```python
from build123d import *

# Parameters (mm, degrees)
SKETCH1_W                        = 287
SKETCH1_H                        = 303
BOSS_EXTRUDE1_DEPTH              = 1.5
SKETCH8_W                        = 1.5
SKETCH8_H                        = 303
BOSS_EXTRUDE8_DEPTH              = 20
BOSS_EXTRUDE12_DEPTH             = 1.5
BOSS_EXTRUDE13_DEPTH             = 1.5
BOSS_EXTRUDE14_REACH             = 217.497
BOSS_EXTRUDE14_DIRECTION_2_REACH = 217.497


with BuildPart() as part:
    # Sketch1 → Boss-Extrude1 (new body)
    with BuildSketch(Plane(origin=(0, 0, 0), x_dir=(1, 0, 0), z_dir=(0, 1, 0))):
        Rectangle(SKETCH1_W, SKETCH1_H)
    extrude(amount=BOSS_EXTRUDE1_DEPTH)

    # Sketch8 → Boss-Extrude8 (add)
    with BuildSketch(Plane(origin=(0, 1.5, 0), x_dir=(1, 0, 0), z_dir=(0, 1, 0))):
        with Locations((-142.75, 0)):
            Rectangle(SKETCH8_W, SKETCH8_H)
        with Locations((142.75, 0)):
            Rectangle(SKETCH8_W, SKETCH8_H)
    extrude(amount=BOSS_EXTRUDE8_DEPTH)

    # Sketch12 → Boss-Extrude12 (add)
    with BuildSketch(Plane.ZY.offset(143.5)):
        Polygon((-151.5, 21.5), (-159.325360037, 21.5), (-151.5, 0), align=None)
    extrude(amount=-BOSS_EXTRUDE12_DEPTH)

    # Sketch13 → Boss-Extrude13 (add)
    with BuildSketch(Plane(origin=(143.5, 0, 0), x_dir=(0, 0, -1), z_dir=(1, 0, 0))):
        Polygon((151.5, 0), (151.5, 21.5), (159.325360037, 21.5), align=None)
    extrude(amount=-BOSS_EXTRUDE13_DEPTH)

    # Boss-Extrude14: up to this face of the body (flat: up to its plane)
    boss_extrude14_end = Plane(part.part.faces().sort_by_distance((142, 11.538792752, -2.109985057))[0])
    # Sketch15 → Boss-Extrude14 (add, up to the picked face)
    with BuildSketch(Plane(origin=(0, 0, 0), x_dir=(0, 0, -1), z_dir=(1, 0, 0)), mode=Mode.PRIVATE) as boss_extrude14_sk1:
        with BuildLine():
            Line((151.5, 1.5), (158.340402867, 20.293852416))
            Line((158.340402867, 20.293852416), (159.749941798, 19.780822201))
            Line((159.749941798, 19.780822201), (152.909538931, 0.986969785))
            ThreePointArc((152.909538931, 0.986969785), (152.360364655, 0.271271934), (151.5, 0))
            Line((151.5, 0), (151.5, 1.5))
        make_face()
    boss_extrude14_tool1 = split(extrude(boss_extrude14_sk1.sketch, amount=BOSS_EXTRUDE14_REACH, mode=Mode.PRIVATE), bisect_by=boss_extrude14_end, keep=Keep.BOTH, mode=Mode.PRIVATE)
    add(boss_extrude14_tool1.solids().sort_by(Axis((0, 10.206295, -155.467858), (1, 0, 0)))[0])

    # Boss-Extrude14 direction 2: up to this face of the body (flat: up to its plane)
    boss_extrude14_direction_2_end = Plane(part.part.faces().sort_by_distance((-142, 11.538792752, -2.109985057))[0])
    # Sketch15 → Boss-Extrude14 direction 2 (add, up to the picked face)
    with BuildSketch(Plane(origin=(0, 0, 0), x_dir=(0, 0, -1), z_dir=(1, 0, 0)), mode=Mode.PRIVATE) as boss_extrude14_direction_2_sk1:
        with BuildLine():
            Line((151.5, 1.5), (158.340402867, 20.293852416))
            Line((158.340402867, 20.293852416), (159.749941798, 19.780822201))
            Line((159.749941798, 19.780822201), (152.909538931, 0.986969785))
            ThreePointArc((152.909538931, 0.986969785), (152.360364655, 0.271271934), (151.5, 0))
            Line((151.5, 0), (151.5, 1.5))
        make_face()
    boss_extrude14_direction_2_tool1 = split(extrude(boss_extrude14_direction_2_sk1.sketch, amount=-BOSS_EXTRUDE14_DIRECTION_2_REACH, mode=Mode.PRIVATE), bisect_by=boss_extrude14_direction_2_end, keep=Keep.BOTH, mode=Mode.PRIVATE)
    add(boss_extrude14_direction_2_tool1.solids().sort_by(Axis((0, 10.206295, -155.467858), (-1, 0, 0)))[0])


solid = part.part
```
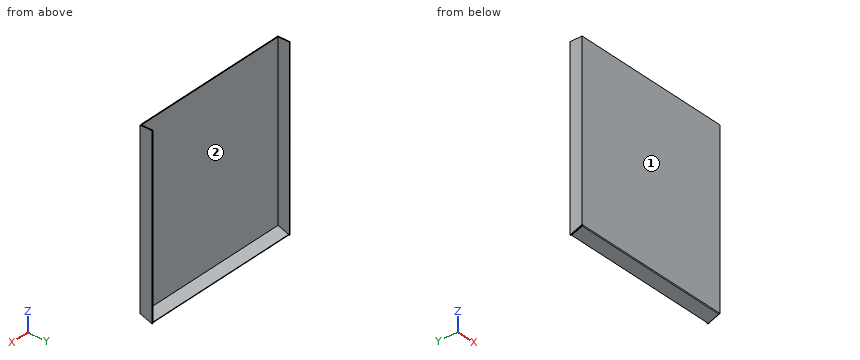
Read the model definition and answer for the solid it produces. Units are mm, in the model's axes. Face numbers are marked on the shaded views. Give positions to 0.01 mm unless a question says otherwise; leave off trailing zeros. Write each loop counter-clockwise with the first axis right and the second up, starting at its lowest first coordinate (ties: lowest second). Pieces come first, ordered by that corner, then holes. Notation, with made-up numbers: (8, 0.5) -> (19, 0.5) arc R21 cw to (19, 32.5) -> close; hole circle Ø5 at (-15.75, 64.25). An arc over 180 degrees is marked (long way). Answer as a JSON object with one key per item and string values.
1) Flat-ended cylindrical pins translate along their axes: pin 1 Ø1 at (x, y) = (-90, 6.5) entering from +Z; pin 2 Ø1.5 at (x, y) = (-101, 15.5) entering from -Z; pin 3 Ø3 at (x, y) = (-34.5, 16) entering from +Z. Find the tip coordinate at first contact, or state that the pin passes through.
Findings below:
{"pin 1": "stops at z = -153.14", "pin 2": "stops at z = -158.46", "pin 3": "stops at z = -156.23"}
2) Section A-A on x = -120.5 is taken. Write down the section's boundary in (y, z).
Findings below:
{"outline": "(0, -151.5) arc R1.5 ccw to (0.99, -152.91) -> (19.78, -159.75) -> (20.29, -158.34) -> (1.5, -151.5) -> (1.5, 151.5) -> (0, 151.5) -> close"}
3) Section B-B on z = 99 is taken. Write down the section's boundary in (x, y).
Findings below:
{"outline": "(-143.5, 0) -> (143.5, 0) -> (143.5, 21.5) -> (142, 21.5) -> (142, 1.5) -> (-142, 1.5) -> (-142, 21.5) -> (-143.5, 21.5) -> close"}
4) Straight lines are drawn through the part: probe 1 along X at (y, z) = (12.5, 70.5); probe 2 along Y at (x, z) = (-98.5, 90.5); probe 3 along Z at (x, y) = (-123.5, 2.75). For each, find the intervals that lie inside material, in ascending order. Write a range as from..to.
Findings below:
{"probe 1": "x = -143.5..-142, 142..143.5", "probe 2": "y = 0..1.5", "probe 3": "z = -153.55..-151.95"}
5) For a pull along X with two mould halves and no side action, classify the marked faces 1 and 2 as pulls with the +X half, pulls with the -X half, needs draft (parallel to the pull), parting line crosses it, or undercut.
Findings below:
{"face 1": "needs draft", "face 2": "undercut"}
6) Section C-C on y = 7.5 is taken. Write down the section's boundary in (x, z), then the cut area to 3 significant figures.
Findings below:
{"outline": "(-143.5, -154.23) -> (-142, -154.23) -> (-142, -155.28) -> (142, -155.28) -> (142, -154.23) -> (143.5, -154.23) -> (143.5, 151.5) -> (142, 151.5) -> (142, -153.68) -> (-142, -153.68) -> (-142, 151.5) -> (-143.5, 151.5) -> close", "area": "1,370 mm^2"}
